Work out the finished part from the listing and answer in its coordinate system (mm). Face numbers are marked on the shaded views. A direction names the side the tool comes from. Round coordinates to 2 decimals unless told otherwise and drop trailing zeros. Loops run counter-clockwise (first coordinate to the right, second up) from the corner with the lowest first, then second, coordinate; pieces in that order, holes last. Notation, with made-up numbers: (51.25, -40) - (93.25, -40) arc R7 ccw to (93.25, -35) - close; hole circle Ø10 at (26.5, 16.25). An arc over 180 degrees is marked (long way). Use CSV: the item, a comma, the result in double quotes. Start each with the question number.
from build123d import *

# Parameters (mm, degrees)
SKETCH1_W               = 40
SKETCH1_H               = 20
BOSS_EXTRUDE1_DEPTH     = 5
SKETCH2_W               = 4.95
SKETCH2_H               = 15
BOSS_EXTRUDE2_DEPTH     = 16.5
CUT_EXTRUDE1_DEPTH      = 37.311155311
CUT_EXTRUDE1_DEPTH_BACK = 37.311155311
SKETCH3_R               = 3
FILLET1_R               = 7.5
SKETCH4_W               = 5.1
SKETCH4_H               = 15
BOSS_EXTRUDE3_DEPTH     = 1
CHAMFER1_SIZE           = 0.5
FILLET2_R               = 2
CUT_EXTRUDE2_DEPTH      = 28.789386463
CUT_EXTRUDE2_DEPTH_BACK = 28.789386463
SKETCH5_R               = 2
SKETCH7_R               = 3.25
CUT_EXTRUDE3_DEPTH      = 2.5
CHAMFER2_SIZE           = 1


with BuildPart() as part:
    # Sketch1 → Boss-Extrude1 (new body)
    with BuildSketch(Plane.XY):
        Rectangle(SKETCH1_W, SKETCH1_H)
    extrude(amount=BOSS_EXTRUDE1_DEPTH)

    # Sketch2 → Boss-Extrude2 (add)
    with BuildSketch(Plane.XY.offset(5)):
        with Locations((-5.025, 0)):
            Rectangle(SKETCH2_W, SKETCH2_H)
        with Locations((5.025, 0)):
            Rectangle(SKETCH2_W, SKETCH2_H)
    extrude(amount=BOSS_EXTRUDE2_DEPTH)

    # Sketch3 → Cut-Extrude1 (cut, two sides: drawn at the far end of the back side and taken through both)
    with BuildSketch(Plane.ZY.offset(7.5).offset(-CUT_EXTRUDE1_DEPTH_BACK)):
        with Locations(Location((14, 0, 0), (0, 0, 270))):
            Circle(SKETCH3_R)
    extrude(amount=CUT_EXTRUDE1_DEPTH + CUT_EXTRUDE1_DEPTH_BACK, mode=Mode.SUBTRACT)

    # Fillet1
    fillet1_edges = [part.edges().sort_by_distance(p)[0] for p in [
        (5.025, -7.5, 21.5),
        (5.025, 7.5, 21.5),
        (-5.025, -7.5, 21.5),
        (-5.025, 7.5, 21.5),
    ]]
    fillet(fillet1_edges, radius=FILLET1_R - 0.0001)  # a hair under: the kernel refuses the full size

    # Sketch4 → Boss-Extrude3 (add)
    with BuildSketch(Plane.XY.offset(5)):
        Rectangle(SKETCH4_W, SKETCH4_H)
    extrude(amount=BOSS_EXTRUDE3_DEPTH)

    # Chamfer1
    chamfer1_edges = [part.edges().sort_by_distance(p)[0] for p in [
        (0, 7.5, 5),
        (-7.5, 0, 5),
        (0, -7.5, 5),
        (7.5, 0, 5),
        (-7.5, 3, 14),
        (-2.55, 3, 14),
        (2.55, 3, 14),
        (7.5, 3, 14),
        (7.5, 7.5, 9.50005),
        (7.5, -7.5, 9.50005),
        (7.5, 5.303330148, 19.303330148),
        (7.5, -5.303330148, 19.303330148),
        (2.55, -7.5, 10.00005),
        (2.55, 7.5, 10.00005),
        (2.55, 5.303330148, 19.303330148),
        (2.55, -5.303330148, 19.303330148),
        (-2.55, 7.5, 10.00005),
        (-2.55, -7.5, 10.00005),
        (-2.55, 5.303330148, 19.303330148),
        (-2.55, -5.303330148, 19.303330148),
        (-7.5, -7.5, 9.50005),
        (-7.5, 7.5, 9.50005),
        (-7.5, 5.303330148, 19.303330148),
        (-7.5, -5.303330148, 19.303330148),
        (2.55, 0, 6),
        (0, 7.5, 6),
        (-2.55, 0, 6),
        (0, -7.5, 6),
    ]]
    chamfer(chamfer1_edges, length=CHAMFER1_SIZE - 0.0001)  # a hair under: the kernel refuses the full size

    # Fillet2
    fillet2_edges = [part.edges().sort_by_distance(p)[0] for p in [
        (20, 0, 5),
        (0, 10, 5),
        (-20, 0, 5),
        (0, -10, 5),
    ]]
    fillet(fillet2_edges, radius=FILLET2_R)

    # Sketch5 → Cut-Extrude2 (cut, two sides: drawn at the far end of the back side and taken through both)
    with BuildSketch(Plane.XY.offset(5).offset(-CUT_EXTRUDE2_DEPTH_BACK)):
        with Locations((-13, 0)):
            Circle(SKETCH5_R)
        with Locations(Location((13, 0, 0), (0, 0, 180))):
            Circle(SKETCH5_R)
    extrude(amount=CUT_EXTRUDE2_DEPTH + CUT_EXTRUDE2_DEPTH_BACK, mode=Mode.SUBTRACT)

    # Sketch7 → Cut-Extrude3 (cut)
    with BuildSketch(Plane.XY.offset(5)):
        with Locations((-13, 0)):
            Circle(SKETCH7_R)
        with Locations(Location((13, 0, 0), (0, 0, 180))):
            Circle(SKETCH7_R)
    extrude(amount=-CUT_EXTRUDE3_DEPTH, mode=Mode.SUBTRACT)

    # Chamfer2
    chamfer2_edges = [part.edges().sort_by_distance(p)[0] for p in [
        (-16.25, 0, 2.5),
        (16.25, 0, 2.5),
    ]]
    chamfer(chamfer2_edges, length=CHAMFER2_SIZE)


solid = part.part
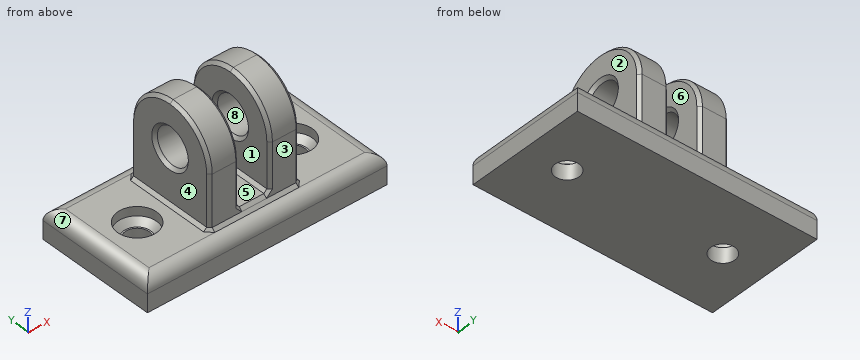
Item 1: Each of these flat-tipped pins is pushed along its axis until it touches: pin 1 Ø5 at (y, z) = (3, 10.5) entering from -X; pin 2 Ø2 at (x, z) = (-4.5, 18.5) entering from -Y; pin 3 Ø4.5 at (x, y) = (0, 0.5) entering from +Z. Where does it stop, or does it pass through?
Item 2: Which of the six approach directions +Z, -Z, +X, -X, +Y, -Y give full straight-line access (tool end or side, diameter ignored) to the marked faces 1, 2, 3 and 4?
Item 3: A cutting plane is placed at A-A (x = 13). Determine the outline of the cut face in (y, z).
Item 4: The mould has two halves that part along X. Classify the marked faces 5, 6, 7 and 8: pulls with the +X half, pulls with the -X half, needs draft (parallel to the pull), parting line crosses it, or undercut.
Item 5: Find the intervals of material crossed by probe 1 along X at (y, z) = (4.5, 16.75); probe 2 along Z at (x, y) = (5, 0); probe 3 along Y at (x, z) = (13, 1.35), in increasing order. Write a range as [from, to].
Result sheet:
1,pin 1,"x = -7.5"
1,pin 2,"y = -6.63"
1,pin 3,"z = 6.2"
2,face 1,"+Z, +Y, -Y"
2,face 2,"+Z, +X, +Y, -Y"
2,face 3,"+Z, +X, -X, -Y"
2,face 4,"+Z, -X, +Y, -Y"
3,outline,"(-10, 0) - (-2, 0) - (-2, 2.5) - (-2.25, 2.5) - (-3.25, 3.5) - (-3.25, 5) - (-8, 5) arc R2 ccw to (-10, 3) - close; (2, 0) - (10, 0) - (10, 3) arc R2 ccw to (8, 5) - (3.25, 5) - (3.25, 3.5) - (2.25, 2.5) - (2, 2.5) - close"
4,face 5,"undercut"
4,face 6,"undercut"
4,face 7,"pulls with the -X half"
4,face 8,"needs draft"
5,probe 1,"[-7.5, -2.55], [2.55, 7.5]"
5,probe 2,"[0, 11], [17, 21.5]"
5,probe 3,"[-10, -2], [2, 10]"
